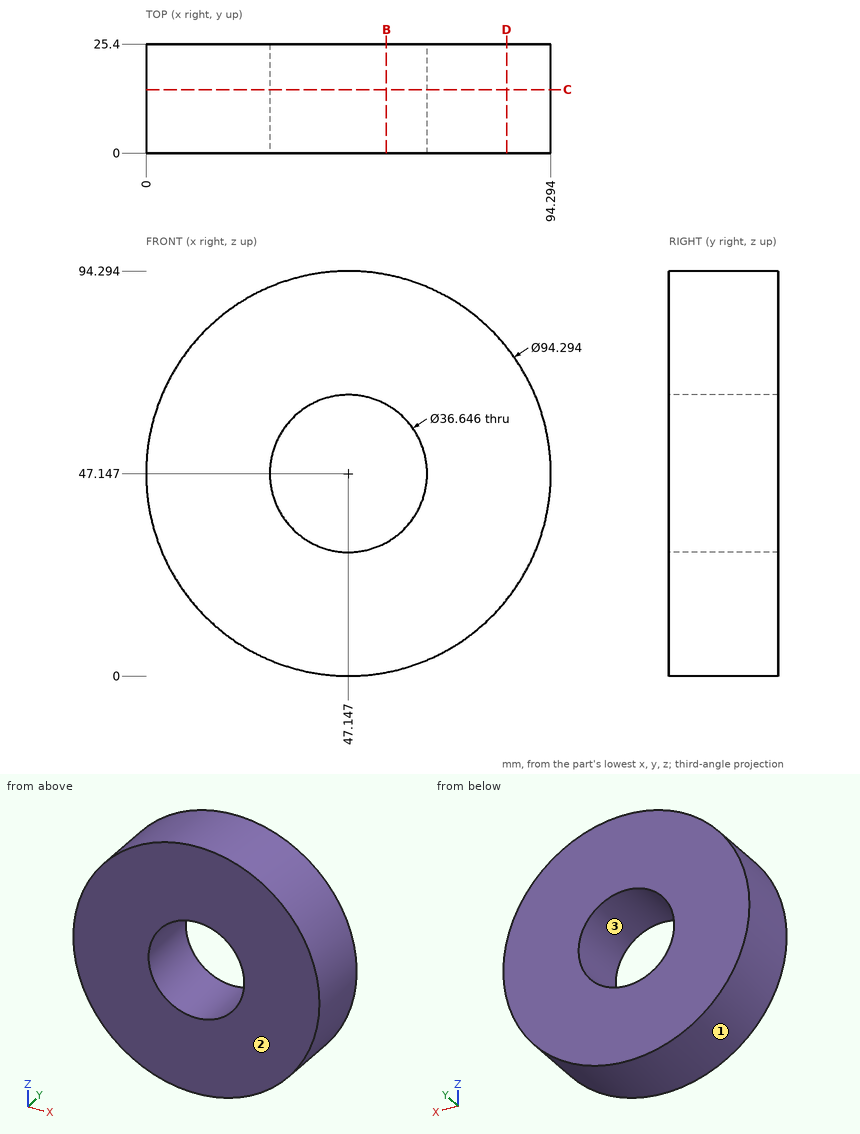
Check sheet for the drawn part. Datum: minimum x, y, z corner. Units: mm. Give positions to 0.01 mm unless a question says otherwise; leave off trailing zeros. Write each loop counter-clockwise with the first axis right and the second up, starting at its lowest first coordinate (ties: lowest second). Pieces come first, ordered by that corner, then holes. Notation, with made-up numbers: (53.5, 3.5) -> (73.5, 3.5) arc R16 cw to (73.5, 17.5) -> close; hole circle Ø11 at (-23.5, 45). An arc over 180 degrees is marked (long way). Use one line per item in the form item = value. Start each with the question number.
1. Thickness scan on line 1 along Z through (x, y) = (47.5, 21.5); line 2 along X through (y, z) = (21.25, 32) (1 decimal); line 3 along Z through (x, y) = (43, 24) (1 decimal). Record the ranges inside material, lowest first. Write a range as from..to.
2. Section check C-C (y = 14.75). Record the cut outline in (x, z) (1 decimal), and give its area (3 significant figures).
3. Section check D-D (x = 84). Record the cut outline in (y, z).
4. Mould release check, pull along Z, two halves, no side actions. Record for the marked faces 1, 2 and 3: pulls with the +Z half, pulls with the -Z half, needs draft (parallel to the pull), parting line crosses it, or undercut.
5. Section check B-B (x = 56). Record the cut outline in (y, z) (1 decimal), and give its area (3 significant figures).
6. Go/stop test with flat-tipped pins: P1, Ø1, axis at y = 16, z = 22.5, coming from the +X side; P2, Ø22, axis at x = 47.15, z = 47.15, coming from the +Y side; P3, Ø3, axis at x = 60.5, y = 17.5, coming from the +Z side; P4, Ø10, axis at y = 13, z = 12, coming from the -X side. Record where each tip stops, or that it passes through.
Conclusion:
q1.line_1 = 0..28.83, 65.47..94.29
q1.line_2 = 2.5..36.8, 57.5..91.8
q1.line_3 = 0.2..29.3, 65..94.1
q2.outline = circle Ø94.3 at (47.1, 47.1); hole circle Ø36.6 at (47.1, 47.1)
q2.area = 5,930 mm²
q3.outline = (0, 17.74) -> (25.4, 17.74) -> (25.4, 76.55) -> (0, 76.55) -> close
q4.face_1 = parting line crosses it
q4.face_2 = needs draft
q4.face_3 = undercut
q5.outline = (0, 0.8) -> (25.4, 0.8) -> (25.4, 31.1) -> (0, 31.1) -> close; (0, 63.2) -> (25.4, 63.2) -> (25.4, 93.5) -> (0, 93.5) -> close
q5.area = 1,540 mm²
q6.P1 = 87.64
q6.P2 = through
q6.P3 = 92.78
q6.P4 = 10.9
